from build123d import *

# Parameters (mm, degrees)
F0_W     = 40
F0_H     = 32
F0_W_2   = 38
F0_H_2   = 30
F1_DEPTH = 5.6
F2_R     = 0.49999


# Not quite as in the source:
# - a fillet or chamfer is up to 0.001 mm smaller than in the source, because OpenCascade refuses the exact size


with BuildPart() as f1:
    # F0 (on Top) → F1 (new body)
    with BuildSketch(Plane.XY):
        Rectangle(F0_W, F0_H)
        Rectangle(F0_W_2, F0_H_2, mode=Mode.SUBTRACT)
    extrude(amount=F1_DEPTH)

    # F2 (radius 0.5 in the source; OpenCascade refuses exactly that, so slightly less here)
    f2_edges = [f1.edges().sort_by_distance(p)[0] for p in [
        (0, 16, 0),
        (-20, 0, 0),
        (0, -16, 0),
        (20, 0, 0),
        (0, 15, 0),
        (19, 0, 0),
        (0, -15, 0),
        (-19, 0, 0),
        (-20, -16, 2.8),
        (20, -16, 2.8),
        (-20, 16, 2.8),
        (20, 16, 2.8),
    ]]
    fillet(f2_edges, radius=F2_R)


solid = f1.part
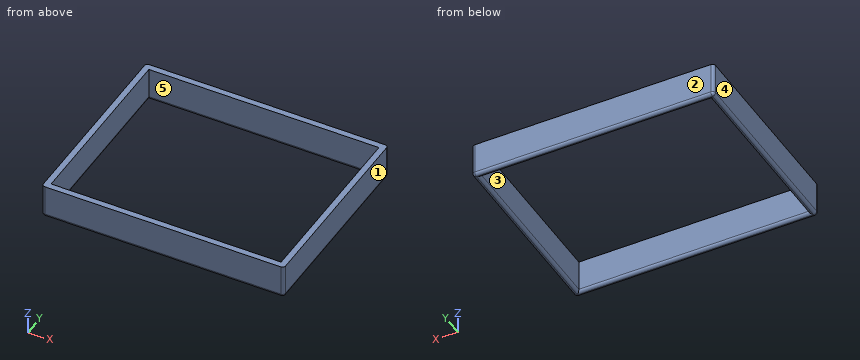
Can you work these out from the model? Positions are in its coordinate system, mm. Face numbers are marked on the shaded views. A direction names the side the tool comes from. Coordinates: 2 decimals unless noted, no trailing zeros. Write each loop counter-clockwise with the first axis right and the second up, starting at its lowest first coordinate (ties: lowest second). Pieces come first, ordered by that corner, then holes. Notation, with made-up numbers: (-36, 25) -> (-13, 25) arc R3 cw to (-13, 30) -> close; hole circle Ø2 at (59.25, 27). An arc over 180 degrees is marked (long way). Write each question's results on one line, items separated by ' | '. Start each with the question number.
Item 1: On a 3-axis mill with a long thin cutter (end or side, diameter ignored), from which of +Z, -Z, +X, -X, +Y, -Y can I reach the whole of each face in a straight line? I mean the marked faces 4 and 5. Say none if no direction works.
Item 2: If we section it at C-C, the plane z = 2.7: Write out the boundary of the cut face in (x, y).
Item 3: Please list where these lines run through material, in increasing order: probe 1 along X at (y, z) = (13, 2.9); probe 2 along Y at (x, z) = (-16.5, 4.75).
Item 4: Thinking about a two-plate mould opening in Y: for the marked faces 1, 2 and 3, which applies, released by +Y, released by -Y, zero draft, split by the parting line, or undercut?
Item 5: I'm going to push a flat-ended pin straight in: P1, Ø10, axis at x = 10, y = 12, coming from the -Z side. Where does the tip first touch, or does it pass through?
Answer block:
1) face 4: +Z, -Z, -X, +Y, -Y | face 5: +Z, -Z
2) outline: (-20, -15.5) arc R0.5 ccw to (-19.5, -16) -> (19.5, -16) arc R0.5 ccw to (20, -15.5) -> (20, 15.5) arc R0.5 ccw to (19.5, 16) -> (-19.5, 16) arc R0.5 ccw to (-20, 15.5) -> close; hole (-19, -15) -> (19, -15) -> (19, 15) -> (-19, 15) -> close
3) probe 1: -20 to -19, 19 to 20 | probe 2: -16 to -15, 15 to 16
4) face 1: zero draft | face 2: released by +Y | face 3: undercut
5) P1: z = 0
